Here's how the part is built. I have some questions about the finished solid (model axes, mm). Round coordinates to 2 decimals unless told otherwise and drop trailing zeros. Order: outer loops, then holes, each group sorted by start corner. A loop starts at its lowest first (then second) coordinate and runs counter-clockwise, first axis right, second up. Notation, with made-up numbers: (-22.5, 77) -> (27.5, 77) arc R20 cw to (27.5, 95) -> close; hole circle Ø7 at (71, 68.25). An arc over 180 degrees is marked (long way). Answer in a Markdown table with one row per item.
```python
from build123d import *

# Parameters (mm, degrees)
F3_R     = 1
F4_DEPTH = 100
F7_W     = 12.659744
F7_H     = 36.118894
F8_DEPTH = 118.783902


with BuildPart() as f2:
    # F0 (on Top) → F2 (revolve)
    with BuildSketch(Plane.XY):
        with BuildLine():
            ThreePointArc((-55.291078, 0), (0, 55.291078), (55.291078, 0))
            Line((55.291078, 0), (59.391451, 0))
            ThreePointArc((59.391451, 0), (0, 59.391451), (-59.391451, 0))
            Line((-59.391451, 0), (-55.291078, 0))
        make_face()
    revolve(axis=Axis((34.508616, 0, 0), (1, 0, 0)))


with BuildPart() as f4:
    # F3 (on Top) → F4 (new body, symmetric)
    with BuildSketch(Plane.XY):
        Circle(F3_R)
    extrude(amount=F4_DEPTH, both=True)


with BuildPart() as f2_1:
    add(f2.part)

    # F5: cut F4
    add(f4.part, mode=Mode.SUBTRACT)

    # F7 (on plane+point) → F8 (cut, through all)
    with BuildSketch(Plane.YZ.offset(59.391451)):
        Rectangle(F7_W, F7_H)
    extrude(amount=-F8_DEPTH, mode=Mode.SUBTRACT)


solid = f2_1.part
```
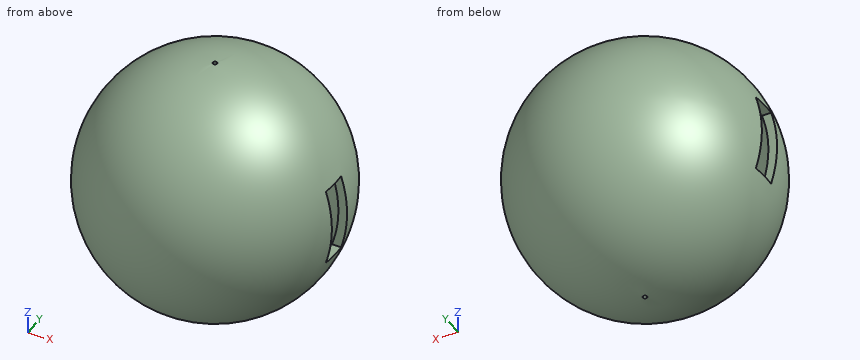
1. Suppose I cut it at C-C on x = 9.5. Write out the boundary of the cut face in (y, z), then the cut area to 3 significant figures.
Numbers:
| item | result |
|---|---|
| outline | circle Ø117.25 at (0, 0); hole circle Ø108.94 at (0, 0) |
| area | 1,480 mm2 |
2. Suppose I cut it at D-D on z = -47.5. Write out the boundary of the cut face in (x, y), then the cut area to 3 significant figures.
Numbers:
| item | result |
|---|---|
| outline | circle Ø71.3 at (0, 0); hole circle Ø56.6 at (0, 0) |
| area | 1,480 mm2 |
3. Suppose I cut it at B-B on y = -3. Write out the boundary of the cut face in (x, z).
Numbers:
| item | result |
|---|---|
| outline | (-56.5, -18.06) arc R59.32 ccw to (56.5, -18.06) -> (52.17, -18.06) arc R55.21 cw to (-52.17, -18.06) -> close; (-56.5, 18.06) -> (-52.17, 18.06) arc R55.21 cw to (52.17, 18.06) -> (56.5, 18.06) arc R59.32 ccw to start |
4. For pin 1 Ø5 at (x, y) = (-55, 0) entering from +Z; pin 2 Ø8 at (x, z) = (55, 6) entering from +Y; pin 3 Ø5.5 at (x, z) = (-55, -5.5) entering from +Y, each with a flat end and sliding along its axis, tell me the tip position at first contact or that it passes through.
Numbers:
| item | result |
|---|---|
| pin 1 | stops at z = 27.77 |
| pin 2 | stops at y = 29.88 |
| pin 3 | stops at y = 27.72 |
5. Please list where these lines run through material, in increasing order: line 1 along Y through (x, z) = (-18, -21.5); line 2 along Z through (x, y) = (-38, 24.5); line 3 along Z through (x, y) = (-44, -7).
Numbers:
| item | result |
|---|---|
| line 1 | y = -52.36 to -47.65, 47.65 to 52.36 |
| line 2 | z = -38.51 to -31.83, 31.83 to 38.51 |
| line 3 | z = -39.27 to -32.74, 32.74 to 39.27 |
6. Suppose I cut it at A-A on z = -2.5. Write out the boundary of the cut face in (x, y).
Numbers:
| item | result |
|---|---|
| outline | (-59, -6.33) arc R59.34 ccw to (59, -6.33) -> (54.87, -6.33) arc R55.23 cw to (-54.87, -6.33) -> close; (-59, 6.33) -> (-54.87, 6.33) arc R55.23 cw to (54.87, 6.33) -> (59, 6.33) arc R59.34 ccw to start |
